from build123d import *

# Parameters (mm, degrees)
F0_R        = 8.001
F0_R_2      = 2.5019
F1_DEPTH    = 5.0038
F2_R        = 6.7818
F2_R_2      = 4.2672
F1_FACE_R   = 8.001
F1_FACE_R_2 = 2.5019
F3_DEPTH    = 0.0508
F4_R        = 6.7818
F4_R_2      = 4.2672
F5_DEPTH    = 0.0508
F6_R        = 0.2032


with BuildPart() as f1:
    # F0 (on Front) → F1 (new body)
    with BuildSketch(Plane.XZ):
        Circle(F0_R)
        Circle(F0_R_2, mode=Mode.SUBTRACT)
    extrude(amount=F1_DEPTH)

    # F2 (on Front) + F1_face (on face) → F3 (cut)
    with BuildSketch(Plane.XZ):
        Circle(F2_R)
        Circle(F2_R_2, mode=Mode.SUBTRACT)
    with BuildSketch(Plane.XZ.offset(5.0038)):
        Circle(F1_FACE_R)
        Circle(F1_FACE_R_2, mode=Mode.SUBTRACT)
    extrude(amount=F3_DEPTH, mode=Mode.SUBTRACT)

    # F4 (on face) → F5 (cut)
    with BuildSketch(Plane.XZ.offset(5.0038)):
        Circle(F4_R)
        Circle(F4_R_2, mode=Mode.SUBTRACT)
    extrude(amount=-F5_DEPTH, mode=Mode.SUBTRACT)

    # F6
    f6_edges = [f1.edges().sort_by_distance(p)[0] for p in [
        (-8.001, -5.0038, 0),
        (-8.001, 0, 0),
    ]]
    fillet(f6_edges, radius=F6_R)


solid = f1.part
Could you check a few things on this model? Use its own coordinates, in mm. A direction names the side the tool comes from. Give positions to 0.01 mm unless a question says otherwise; leave off trailing zeros. Order: outer loops, then holes, each group sorted by start corner. A loop starts at its lowest first (then second) coordinate and runs counter-clockwise, first axis right, second up. Notation, with made-up numbers: (21.25, 55.5) - (70.25, 55.5) arc R8 cw to (70.25, 65.5) - close; hole circle Ø8 at (46, 85). An arc over 180 degrees is marked (long way). One line per item, written item: value. Start each with the question number.
1. For faces 1 (the face through (-0.09, -0.051, -4.43)), 2 (the face through (-6, 0, 4)), which set-ups out of +Z, -Z, +X, -X, +Y, -Y let a thin tool reach every point of the face, with its end or its side?
2. Thinking about a two-plate mould opening in X: for faces 3 (the face through (-0.09, -4.953, -4.43)), 4 (the face through (-2, -2.5, -1.5)), 5 (the face through (-1.73, -2.47, -7.81)), 6 (the face through (2, 0, -2)), which applies, +X half, -X half, draft (parallel to the pull), parting line (faces both ways), or undercut?
3. Imagine slicing it at A-A on z = 0. List the corners of the cut face in (x, y) for me.
4. If I drill on probe 1 along Z at (x, y) = (0, -2.3); probe 2 along Y at (x, z) = (5.75, 0); probe 3 along X at (y, z) = (-2.3, -2.25), over which ranges is the centre line in solid material (lowest first)?
5. Imagine slicing it at C-C on y = -2.3. List the corners of the cut face in (x, z) for me.
6. Imagine slicing it at B-B on x = 0. List the corners of the cut face in (y, z) for me, plus the area to 3 significant figures.
7. For P1, Ø1, axis at y = -2.5, z = 4.5, coming from the -X side; P2, Ø2, axis at x = 1.5, z = -1.5, coming from the -Y side; P3, Ø1, axis at y = -2, z = -5.5, coming from the -X side; P4, Ø4, axis at x = 0, z = 0, coming from the -Y side, each with a flat end and sliding along its axis, tell me the tip position at first contact or that it passes through.
Values:
1. face 1: +Y
1. face 2: +Z, -Z, +X, -X, +Y
2. face 3: undercut
2. face 4: undercut
2. face 5: parting line
2. face 6: draft
3. outline: (-8, -4.8) arc R0.2 ccw to (-7.8, -5) - (-6.78, -5) - (-6.78, -4.95) - (-4.27, -4.95) - (-4.27, -5) - (-2.5, -5) - (-2.5, 0) - (-4.27, 0) - (-4.27, -0.05) - (-6.78, -0.05) - (-6.78, 0) - (-7.8, 0) arc R0.2 ccw to (-8, -0.2) - close; (2.5, -5) - (4.27, -5) - (4.27, -4.95) - (6.78, -4.95) - (6.78, -5) - (7.8, -5) arc R0.2 ccw to (8, -4.8) - (8, -0.2) arc R0.2 ccw to (7.8, 0) - (6.78, 0) - (6.78, -0.05) - (4.27, -0.05) - (4.27, 0) - (2.5, 0) - close
4. probe 1: -8 to -2.5, 2.5 to 8
4. probe 2: -4.95 to -0.05
4. probe 3: -7.68 to -1.09, 1.09 to 7.68
5. outline: circle Ø16 at (0, 0); hole circle Ø5 at (0, 0)
6. outline: (-5, -7.8) arc R0.2 ccw to (-4.8, -8) - (-0.2, -8) arc R0.2 ccw to (0, -7.8) - (0, -6.78) - (-0.05, -6.78) - (-0.05, -4.27) - (0, -4.27) - (0, -2.5) - (-5, -2.5) - (-5, -4.27) - (-4.95, -4.27) - (-4.95, -6.78) - (-5, -6.78) - close; (-5, 2.5) - (0, 2.5) - (0, 4.27) - (-0.05, 4.27) - (-0.05, 6.78) - (0, 6.78) - (0, 7.8) arc R0.2 ccw to (-0.2, 8) - (-4.8, 8) arc R0.2 ccw to (-5, 7.8) - (-5, 6.78) - (-4.95, 6.78) - (-4.95, 4.27) - (-5, 4.27) - close
6. area: 54.5 mm²
7. P1: x = -6.93
7. P2: y = -5
7. P3: x = -6.25
7. P4: through
